from build123d import *

# Parameters (mm, degrees)
F0_W         = 4
F0_H         = 51
F0_H_2       = 4
F0_W_2       = 21
F1_DEPTH     = 15
F4_D         = 3.5
F4_ON_F3_D   = 3.5
F5_DEPTH     = 25
F6_DEPTH     = 25
F7_T1_DEPTH  = 4
F7_T3_DEPTH  = 14
F7_T5_DEPTH  = 13.3694414049
F7_T7_DEPTH  = 14
F7_T9_DEPTH  = 30.9469097591
F7_T11_DEPTH = 13.6920837807


# Not quite as in the source:
# - a fillet or chamfer that OpenCascade refuses, or shapes differently, is made with other operations: its cross-section is extruded or revolved along the edge and cut away or added


with BuildPart() as f1:
    # F0 (on Top) → F1 (new body)
    with BuildSketch(Plane.XY):
        with Locations((0, 2)):
            Rectangle(F0_W, F0_H)
        with Locations((0, -25.5)):
            Rectangle(F0_W, F0_H_2)
        with Locations((12.5, -25.5)):
            Rectangle(F0_W_2, F0_H_2)
    extrude(amount=F1_DEPTH)

    # F4 (through all)
    with Locations(Plane(origin=(-2, 0, 0), x_dir=(0, -1, 0), z_dir=(-1, 0, 0))):
        with Locations((-23.34, 5.4024579003), (7.7, 5.4024579003)):
            Hole(F4_D / 2)

    # F4 on F3 (through all)
    with Locations(Plane.XZ.offset(27.5)):
        with Locations((18, 8.8024579003)):
            Hole(F4_ON_F3_D / 2)

    # F2 (on face) → F5 (cut)
    with BuildSketch(Plane(origin=(-2, 0, 0), x_dir=(0, -1, 0), z_dir=(-1, 0, 0))):
        Polygon((-27.5, 15), (-27.5, 10.3389231786), (21.5976021229, 10.3389231786), (24.1305585951, 15), align=None)
    extrude(amount=-F5_DEPTH, mode=Mode.SUBTRACT)

    # F3 (on face) → F6 (cut)
    with BuildSketch(Plane.XZ.offset(27.5)):
        Polygon((23, 0), (23, 4), (9.7110802308, 4), (1.6920837807, 0), align=None)
    extrude(amount=-F6_DEPTH, mode=Mode.SUBTRACT)

    # F7: fillet of radius 2 on 7 edges, made by hand

    # F7_s2 → F7_t1 (join)
    with BuildSketch(Plane.XZ.offset(23.5)):
        with BuildLine():
            ThreePointArc((9.2894845277, 3.7897015141), (9.7236323162, 3.9467155709), (10.1822154449, 4))
            Line((10.1822154449, 4), (9.7110802308, 4))
            Line((9.7110802308, 4), (9.2894845277, 3.7897015141))
        make_face()
    extrude(amount=F7_T1_DEPTH)

    # F7_s4 → F7_t3 (cut)
    with BuildSketch(Plane.YZ.offset(-7)):
        with BuildLine():
            ThreePointArc((27.5, 8.3389231786), (26.9142135624, 9.753136741), (25.5, 10.3389231786))
            Line((25.5, 10.3389231786), (27.5, 10.3389231786))
            Line((27.5, 10.3389231786), (27.5, 8.3389231786))
        make_face()
        with BuildLine():
            ThreePointArc((27.5, 2), (26.9142135624, 0.5857864376), (25.5, 0))
            Line((25.5, 0), (27.5, 0))
            Line((27.5, 0), (27.5, 2))
        make_face()
    extrude(amount=F7_T3_DEPTH, mode=Mode.SUBTRACT)

    # F7_s6 → F7_t5 (cut)
    with BuildSketch(Plane.XZ.offset(19.1305585951)):
        with BuildLine():
            ThreePointArc((21, 15), (22.4142135624, 14.4142135624), (23, 13))
            Line((23, 13), (23, 15))
            Line((23, 15), (21, 15))
        make_face()
    extrude(amount=F7_T5_DEPTH, mode=Mode.SUBTRACT)

    # F7_s8 → F7_t7 (cut)
    with BuildSketch(Plane.XZ.offset(18.5)):
        with BuildLine():
            ThreePointArc((21, 4), (22.4142135624, 4.5857864376), (23, 6))
            Line((23, 6), (23, 4))
            Line((23, 4), (21, 4))
        make_face()
    extrude(amount=F7_T7_DEPTH, mode=Mode.SUBTRACT)

    # F7_s10 → F7_t9 (cut)
    with BuildSketch(Plane.YZ.offset(-4.9734548795)):
        with BuildLine():
            ThreePointArc((-25.3199405469, 15), (-24.2976673595, 14.7189989908), (-23.5626539694, 13.9549575303))
            Line((-23.5626539694, 13.9549575303), (-24.1305585951, 15))
            Line((-24.1305585951, 15), (-25.3199405469, 15))
        make_face()
    extrude(amount=F7_T9_DEPTH, mode=Mode.SUBTRACT)

    # F7_s12 → F7_t11 (cut)
    with BuildSketch(Plane.YZ.offset(-7)):
        with BuildLine():
            ThreePointArc((-25.5, 0), (-26.9142135624, 0.5857864376), (-27.5, 2))
            Line((-27.5, 2), (-27.5, 0))
            Line((-27.5, 0), (-25.5, 0))
        make_face()
    extrude(amount=F7_T11_DEPTH, mode=Mode.SUBTRACT)


solid = f1.part
Check sheet for the modelled part. Datum: model origin and axes. Units: mm. A direction names the side the tool comes from. Give positions to 0.01 mm unless a question says otherwise; leave off trailing zeros. Write each loop counter-clockwise with the first axis right and the second up, starting at its lowest first coordinate (ties: lowest second). Pieces come first, ordered by that corner, then holes. Notation, with made-up numbers: (60, -38.75) -> (74, -38.75) arc R22 cw to (74, -10.75) -> close; hole circle Ø5 at (36, -20.5). An arc over 180 degrees is marked (long way). One line per item, written item: value. Start each with the question number.
Item 1: Section check D-D on x = 14.5. Record the cut outline in (y, z).
Item 2: Section check C-C on z = 9.75. Record the cut outline in (x, y), then the cut area to 3 significant figures.
Item 3: Section check A-A on y = -7.7. Record the cut outline in (x, z), then the cut area to 3 significant figures.
Item 4: Draft check along X on faces 6 (the cylindrical face through (22.4, -25.47, 4.57)), 7 (the cylindrical face through (19.39, -25.47, 7.74)), 8 (the cylindrical face through (10.205, -24.311, 14.727)), 9 (the flat face through (-2, 0, 6)). Enter one of: +X half, -X half, draft (parallel to the pull), parting line (faces both ways), or undercut.
Item 5: Tool access check on faces 1 (the flat face through (16, -26, 4)), 2 (the flat face through (4.9, -24.3, 1.6)), 3 (the flat face through (2, 2, 5)), 4 (the flat face through (0, 2, 10.339)), 5 (the flat face through (23, -26, 9)). Record the directions out of +Z, -Z, +X, -X, +Y, -Y that give a thin tool (end or side, any length) a straight path to the whole face; none if there is none.
Item 6: Gauge pin test, flat ends, axial feed: pin 1 (4.5 mm diameter, centred on x = 13.5, y = -25.5, fed in from -Z); pin 2 (1 mm diameter, centred on x = 6, z = 2, fed in from +Y); pin 3 (5.5 mm diameter, centred on y = 23.34, z = 5.4, fed in from +X). Record the tip position at first contact, or that the pin passes through.
Item 7: Material ranges on probe 1 along Z at (x, y) = (-0.4, -7.7); probe 2 along Z at (x, y) = (18, -25.7); probe 3 along X at (y, z) = (-16.5, 5.25), recorded low to high. Write a range as from..to.
Item 8: Section check B-B on x = 18. Record the cut outline in (y, z).
Results list:
1. outline: (-27.5, 4) -> (-23.5, 4) -> (-23.5, 13.84) -> (-23.56, 13.95) arc R2 ccw to (-25.32, 15) -> (-27.5, 15) -> close
2. outline: (-2, -27.5) -> (16.53, -27.5) -> (16.53, -23.5) -> (2, -23.5) -> (2, 26.92) -> (-2, 26.92) -> close; (19.47, -27.5) -> (23, -27.5) -> (23, -23.5) -> (19.47, -23.5) -> close
2. area: 290 mm²
3. outline: (-2, 0) -> (1.69, 0) -> (2, 0.15) -> (2, 3.65) -> (-2, 3.65) -> close; (-2, 7.15) -> (2, 7.15) -> (2, 10.34) -> (-2, 10.34) -> close
3. area: 27.3 mm²
4. face 6: +X half
4. face 7: undercut
4. face 8: draft
4. face 9: -X half
5. face 1: -Z, +X, +Y, -Y
5. face 2: -Z, +X, -Y
5. face 3: +Z, -Z, +X, +Y
5. face 4: +Z, +X, -X, +Y
5. face 5: +Z, -Z, +X, +Y, -Y
6. pin 1: z = 4
6. pin 2: y = -23.5
6. pin 3: x = 2
7. probe 1: 0..3.65, 7.15..10.34
7. probe 2: 4..7.05, 10.55..15
7. probe 3: -2..2
8. outline: (-27.5, 4) -> (-23.5, 4) -> (-23.5, 7.05) -> (-27.5, 7.05) -> close; (-27.5, 10.55) -> (-23.5, 10.55) -> (-23.5, 13.84) -> (-23.56, 13.95) arc R2 ccw to (-25.32, 15) -> (-27.5, 15) -> close
